Can you work these out from the drawing? Everything is in mm from the part's minimum corner. A direction names the side the tool comes from. Give positions to 0.01 mm unless a question says otherwise; leave off trailing zeros. Write each loop counter-clockwise with the first axis right and the second up, starting at its lowest first coordinate (ties: lowest second). Pieces come first, ordered by that corner, then holes. Notation, with made-up numbers: (-7.5, 48.25) -> (21.5, 48.25) arc R10 cw to (21.5, 56.25) -> close; hole circle Ø3 at (-24, 38). An arc over 180 degrees is marked (long way). Use one line per item in the form item = value.
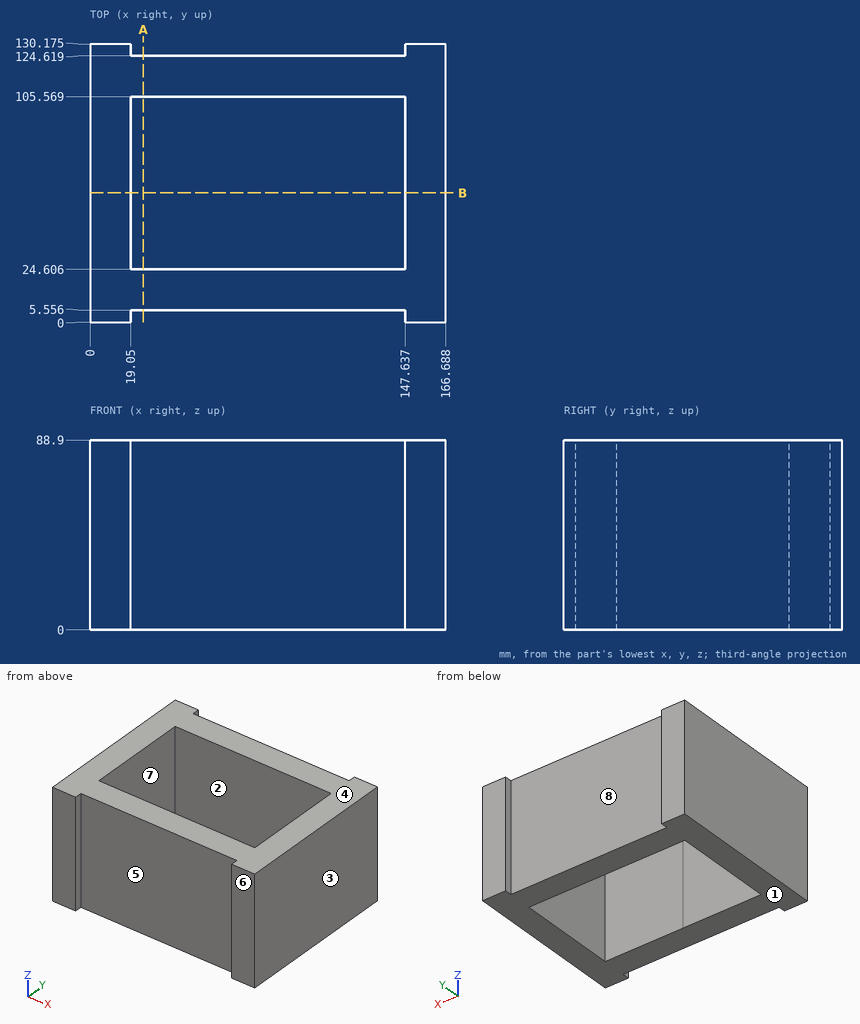
Q1. Which directions (+Z, -Z, +X, -X, +Y, -Y) give clear straight access to the entire face, cutting with the end or side of a thin tool? Please do the marked faces 4, 5, 6, 7 and 8.
Result set:
face_4 = +Z, +X, -X, +Y, -Y
face_5 = +Z, -Z, -Y
face_6 = +Z, -Z, +X, -X, -Y
face_7 = +Z, -Z
face_8 = +Z, -Z, +Y
Q2. I want a section at B-B, the plane y = 60.5. Write out the boundary of the cut face in (x, z), and give its area (3 significant figures).
Result set:
outline = (0, 0) -> (19.05, 0) -> (19.05, 88.9) -> (0, 88.9) -> close; (147.64, 0) -> (166.69, 0) -> (166.69, 88.9) -> (147.64, 88.9) -> close
area = 3,390 mm2
Q3. I want a section at A-A, the plane x = 25. Write out the boundary of the cut face in (y, z), and give its area (3 significant figures).
Result set:
outline = (5.56, 0) -> (24.61, 0) -> (24.61, 88.9) -> (5.56, 88.9) -> close; (105.57, 0) -> (124.62, 0) -> (124.62, 88.9) -> (105.57, 88.9) -> close
area = 3,390 mm2
Q4. Will these pins go through, and if not, where does the flat tip stop? pin 1 Ø4.5 at (y, z) = (128, 55) entering from -X; pin 2 Ø19.5 at (x, z) = (112.5, 29) entering from +Y.
Result set:
pin_1 = 0
pin_2 = 124.62
Q5. If we mould it in two halves opening along X, with no side actions, what happens to the marked faces 1, 2 and 3? For each: +X half, -X half, draft (parallel to the pull), parting line (faces both ways), or undercut.
Result set:
face_1 = draft
face_2 = undercut
face_3 = +X half
Q6. If I drill on line 1 along X through (y, z) = (30, 74); line 2 along Y through (x, z) = (91, 77), over which ranges is the centre line in solid material (lowest first)? Write a range as from..to.
Result set:
line_1 = 0..19.05, 147.64..166.69
line_2 = 5.56..24.61, 105.57..124.62
